Part model, mm, in its own coordinate system. A direction names the side the tool comes from. Round coordinates to 2 decimals unless told otherwise and drop trailing zeros. Loops run counter-clockwise (first coordinate to the right, second up) from the corner with the lowest first, then second, coordinate; pieces in that order, holes last. Notation, with made-up numbers: (66.25, -11) - (72.25, -11) arc R14 ccw to (72.25, 7) - close; hole circle Ø5 at (27, -38.5). An arc over 180 degrees is marked (long way). Write each question's results on one line, items separated by ' | '. Start each with the question number.
(1) Mould opens along X. For faces 4 (the face through (0, 7, -1)), 5 (the face through (0, 0, 0)), 6 (the face through (2.685, 7.282, 0.596)) say: released by +X, released by -X, zero draft, split by the parting line, or undercut.
(2) Flat gauge pins, fed straight in: P1, Ø3, axis at y = 5, z = 1.5, coming from the -X side; P2, Ø1, axis at x = 1, y = 3, coming from the +Z side; P3, Ø2, axis at x = -0.5, y = 5.5, coming from the -Z side. Where does each tip first touch, or does it go through?
(3) Tool access for faces 1 (the face through (0.86, 7.03, 0.51)), 2 (the face through (1, 9, -1)), 3 (the face through (1.2, 6, -1.2)): list every direction of +Z, -Z, +X, -X, +Y, -Y with a clear straight run to the whole face (end or side of a thin tool).
(4) Cut at C-C, the plane y = 4.75. List the corners of the cut face in (x, z), then the cut area to 3 significant figures.
(5) Cut at A-A, the plane y = 5.75. List the corners of the cut face in (x, z).
(6) Drill centre lines: L1, parallel to X at y = 8.5, z = 0.15; L2, parallel to Y at x = -0.15, z = 0.4; L3, parallel to Z at x = -0.85, y = 6.25. Where is each one in solid material? Low to high.
(7) Cut at B-B, the plane x = 0. List the corners of the cut face in (y, z), then the cut area to 3 significant figures.
from build123d import *

# Parameters (mm, degrees)
CHAMFER1_SIZE      = 0.4
CUT_EXTRUDE2_DEPTH = 4


with BuildPart() as part:
    # Sketch2 → Revolve1 (revolve)
    with BuildSketch(Plane.XY, mode=Mode.PRIVATE) as revolve1_sk:
        Polygon((0, 9), (2.75, 9), (2.75, 6), (1.5, 6), (1.5, 0), (0, 0), align=None)
    revolve(revolve1_sk.sketch.rotate(Axis((0, 0, 0), (0, 1, 0)), 90), axis=Axis((0, 0, 0), (0, 1, 0)))

    # Chamfer1
    chamfer1_edges = [part.edges().sort_by_distance(p)[0] for p in [
        (0, 0, 1.5),
        (0, 9, 2.75),
    ]]
    chamfer(chamfer1_edges, length=CHAMFER1_SIZE)

    # Sketch4 → Cut-Extrude2 (cut)
    with BuildSketch(Plane(origin=(0, 9, 0), x_dir=(1, 0, 0), z_dir=(0, 1, 0))):
        Polygon((1.154700538, 0), (0.577350269, 1), (-0.577350269, 1), (-1.154700538, 0), (-0.577350269, -1), (0.577350269, -1), align=None)
    extrude(amount=-CUT_EXTRUDE2_DEPTH, mode=Mode.SUBTRACT)


solid = part.part
A:
1) face 4: undercut | face 5: zero draft | face 6: split by the parting line
2) P1: x = -2.72 | P2: z = 1.41 | P3: z = -2.75
3) face 1: +Y | face 2: +Z, -Z, +X, -X, +Y | face 3: -Y
4) outline: circle Ø3 at (0, 0) | area: 7.07 mm2
5) outline: circle Ø3 at (0, 0); hole (-1.15, 0) - (-0.58, -1) - (0.58, -1) - (1.15, 0) - (0.58, 1) - (-0.58, 1) - close
6) L1: -2.75 to -1.07, 1.07 to 2.75 | L2: 0 to 5 | L3: -2.62 to -0.53, 0.53 to 2.62
7) outline: (0, -1.1) - (0.4, -1.5) - (6, -1.5) - (6, -2.75) - (8.6, -2.75) - (9, -2.35) - (9, -1) - (5, -1) - (5, 1) - (9, 1) - (9, 2.35) - (8.6, 2.75) - (6, 2.75) - (6, 1.5) - (0.4, 1.5) - (0, 1.1) - close | area: 26.2 mm2
